```python
from build123d import *

# Parameters (mm, degrees)
F1_DEPTH = 76.2
F2_W     = 28.575
F2_H     = 23.576327
F3_DEPTH = 50.801
F6_D     = 9.398
F8_D     = 9.398
F10_D    = 9.398


with BuildPart() as f1:
    # F0 (on Right) → F1 (new body)
    with BuildSketch(Plane.YZ):
        Polygon((-44.545047, -32.283712), (50.704953, -32.283712), (50.704953, -13.233712), (6.254953, -13.233712), (6.254953, 37.566288), (-19.145047, 37.566288), (-19.145047, -13.233712), (-44.545047, -13.233712), align=None)
    extrude(amount=F1_DEPTH)

    # F2 (on face) → F3 (cut, through all)
    with BuildSketch(Plane(origin=(0, 6.254953, 0), x_dir=(-1, 0, 0), z_dir=(0, 1, 0))):
        with Locations((-38.1, 25.778125)):
            Rectangle(F2_W, F2_H)
    extrude(amount=-F3_DEPTH, mode=Mode.SUBTRACT)

    # F6 (through all)
    with Locations(Plane.XY.offset(-13.233712)):
        with Locations((12.7, 37.945128)):
            Hole(F6_D / 2)

    # F8 (through all)
    with Locations(Plane.XY.offset(-13.233712)):
        with Locations((62.49947, 38.197309)):
            Hole(F8_D / 2)

    # F10 (through all)
    with Locations(Plane.XY.offset(-13.233712)):
        with Locations((12.7, -31.845047), (63.5, -31.845047)):
            Hole(F10_D / 2)


solid = f1.part
```
Part model, mm, in its own coordinate system. A direction names the side the tool comes from. Round coordinates to 2 decimals unless told otherwise and drop trailing zeros. Write each loop counter-clockwise with the first axis right and the second up, starting at its lowest first coordinate (ties: lowest second). Pieces come first, ordered by that corner, then holes.
Item 1: Cut at B-B, the plane x = 12.7. Give the cut face in (y, z), plus the area to 3 significant figures.
Results:
outline: (-44.55, -32.28) - (-36.54, -32.28) - (-36.54, -13.23) - (-44.55, -13.23) - close; (-27.15, -32.28) - (33.25, -32.28) - (33.25, -13.23) - (6.25, -13.23) - (6.25, 37.57) - (-19.15, 37.57) - (-19.15, -13.23) - (-27.15, -13.23) - close; (42.64, -32.28) - (50.7, -32.28) - (50.7, -13.23) - (42.64, -13.23) - close
area: 2,750 mm2
Item 2: Probe L1, parallel to Y at x = 12, z = -27; L2, parallel to X at y = 1.5, z = 29.5; L3, parallel to Y at x = 63.5, z = -24.25. List the from-to ranges inside material, lowest first.
Results:
L1: y = -44.55 to -36.49, -27.2 to 33.3, 42.59 to 50.7
L2: x = 0 to 23.81, 52.39 to 76.2
L3: y = -44.55 to -36.54, -27.15 to 33.61, 42.79 to 50.7
Item 3: Which spindle directions (+Z, -Z, +X, -X, +Y, -Y) get a long thin tool onto all of the face, cutting with end or side? Do faces 5 (the flat face through (38, -19.145, 13)), 6 (the cylindrical face through (61.332, -36.014, -22.892)), 7 (the flat face through (52.388, -6, 26)), 8 (the flat face through (38, 29, -13.234)), 9 (the flat face through (38, 2, -32.284)). Say none if no direction does.
Results:
face 5: +Z, +X, -X, -Y
face 6: +Z, -Z
face 7: +Z, +Y, -Y
face 8: +Z, +X, -X, +Y
face 9: -Z, +X, -X, +Y, -Y
Item 4: Cut at C-C, the plane x = 50.5. Give the cut face in (y, z).
Results:
outline: (-44.55, -32.28) - (50.7, -32.28) - (50.7, -13.23) - (6.25, -13.23) - (6.25, 13.99) - (-19.15, 13.99) - (-19.15, -13.23) - (-44.55, -13.23) - close
Item 5: Two-plate mould, pull along X, no slides. Class faces 1 (the cylindrical face through (63.52, 33.61, -22.89)), 2 (the flat face through (0, -8, -5)), 3 (the flat face through (38, -6, 13.99)), 4 (the flat face through (12, -6, 37.566)): +X half, -X half, draft (parallel to the pull), parting line (faces both ways), or undercut.
Results:
face 1: undercut
face 2: -X half
face 3: undercut
face 4: draft
Item 6: Cut at D-D, the plane z = -21.5. Give the cut face in (x, y).
Results:
outline: (0, -44.55) - (76.2, -44.55) - (76.2, 50.7) - (0, 50.7) - close; hole circle Ø9.4 at (12.7, -31.85); hole circle Ø9.4 at (12.7, 37.95); hole circle Ø9.4 at (62.5, 38.2); hole circle Ø9.4 at (63.5, -31.85)
Item 7: Drop flat-ended pins along their axis: pin 1 Ø5 at (x, z) = (12, 4.5) entering from -Y; pin 2 Ø7.5 at (x, y) = (12.7, -31.85) entering from +Z; pin 3 Ø10 at (x, y) = (35, 39.5) entering from +Z; pin 4 Ø6 at (x, z) = (57, 24.5) entering from +Y. Give the stop position or say it passes through.
Results:
pin 1: stops at y = -19.15
pin 2: passes through
pin 3: stops at z = -13.23
pin 4: stops at y = 6.25
Item 8: Cut at A-A, the plane z = 31. Give the cut face in (x, y), plus the area to 3 significant figures.
Results:
outline: (0, -19.15) - (23.81, -19.15) - (23.81, 6.25) - (0, 6.25) - close; (52.39, -19.15) - (76.2, -19.15) - (76.2, 6.25) - (52.39, 6.25) - close
area: 1,210 mm2
